```python
from build123d import *

# Parameters (mm, degrees)
SKETCH_1_W          = 80
SKETCH_1_H          = 80
EXTRUDE_1_DEPTH     = 134
SKETCH_2_R          = 40
EXTRUDE_2_DEPTH     = 1
SKETCH_3_W          = 90
SKETCH_3_H          = 90
EXTRUDE_3_DEPTH     = 10
SKETCH_4_R          = 40
EXTRUDE_4_DEPTH     = 3
SKETCH_5_R          = 20
CUT_EXTRUDE_1_DEPTH = 10
SKETCH_6_R          = 12.5
EXTRUDE_5_DEPTH     = 10
SKETCH_7_R          = 10
EXTRUDE_6_DEPTH     = 27
SKETCH_9_R          = 3.25
CUT_EXTRUDE_2_DEPTH = 10


with BuildPart() as part:
    # 草图1 → 拉伸1 (new body)
    with BuildSketch(Plane.XY):
        with Locations((40, -40)):
            Rectangle(SKETCH_1_W, SKETCH_1_H)
    extrude(amount=EXTRUDE_1_DEPTH)

    # 草图2 → 拉伸2 (add)
    with BuildSketch(Plane.XY.offset(134)):
        with Locations((40, -40)):
            Circle(SKETCH_2_R)
    extrude(amount=EXTRUDE_2_DEPTH)

    # 草图3 → 拉伸3 (add)
    with BuildSketch(Plane.XY.offset(135)):
        with Locations((40, -40)):
            Rectangle(SKETCH_3_W, SKETCH_3_H)
    extrude(amount=EXTRUDE_3_DEPTH)

    # 草图4 → 拉伸4 (add)
    with BuildSketch(Plane.XY.offset(145)):
        with Locations((40, -40)):
            Circle(SKETCH_4_R)
    extrude(amount=EXTRUDE_4_DEPTH)

    # 草图5 → 切除-拉伸1 (cut)
    with BuildSketch(Plane.XY.offset(148)):
        with Locations((40, -40)):
            Circle(SKETCH_5_R)
    extrude(amount=-CUT_EXTRUDE_1_DEPTH, mode=Mode.SUBTRACT)

    # 草图6 → 拉伸5 (add)
    with BuildSketch(Plane.XY.offset(138)):
        with Locations((40, -40)):
            Circle(SKETCH_6_R)
    extrude(amount=EXTRUDE_5_DEPTH)

    # 草图7 → 拉伸6 (add)
    with BuildSketch(Plane.XY.offset(148)):
        with Locations((40, -40)):
            Circle(SKETCH_7_R)
    extrude(amount=EXTRUDE_6_DEPTH)

    # 草图9 → 切除-拉伸2 (cut)
    with BuildSketch(Plane.XY.offset(145)):
        with Locations((75.355339059, -4.644660941)):
            Circle(SKETCH_9_R)
        with Locations((75.355339059, -75.355339059)):
            Circle(SKETCH_9_R)
        with Locations((4.644660941, -75.355339059)):
            Circle(SKETCH_9_R)
        with Locations((4.644660941, -4.644660941)):
            Circle(SKETCH_9_R)
    extrude(amount=-CUT_EXTRUDE_2_DEPTH, mode=Mode.SUBTRACT)


solid = part.part
```
Here's how the part is built. I have some questions about the finished solid (model axes, mm). A direction names the side the tool comes from. Coordinates: 2 decimals unless noted, no trailing zeros. Loops run counter-clockwise (first coordinate to the right, second up) from the corner with the lowest first, then second, coordinate; pieces in that order, holes last. Notation, with made-up numbers: M 32.25,5 L 69.25,5 A19 ccw 69.25,25 Z; hole C 35,75 d4. An arc over 180 degrees is marked long. One line per item, written item: value.
1. Please list where these lines run through material, in increasing order: probe 1 along Y at (x, z) = (40, 142); probe 2 along Z at (x, y) = (79, -67.5); probe 3 along Z at (x, y) = (31.5, -6).
Geometry says:
probe 1: y = -85 to -60, -52.5 to -27.5, -20 to 5
probe 2: z = 0 to 134, 135 to 145
probe 3: z = 0 to 148
2. Imagine slicing it at D-D (y = -69). List the corners of the cut face in (x, z) for me.
Geometry says:
outline: M -5,135 L 12.45,135 L 12.45,134 L 0,134 L 0,0 L 80,0 L 80,134 L 67.55,134 L 67.55,135 L 85,135 L 85,145 L 67.55,145 L 67.55,148 L 12.45,148 L 12.45,145 L -5,145 Z
3. Imagine slicing it at C-C (x = 43). List the corners of the cut face in (y, z) for me.
Geometry says:
outline: M -85,135 L -79.89,135 L -79.89,134 L -80,134 L -80,0 L 0,0 L 0,134 L -0.11,134 L -0.11,135 L 5,135 L 5,145 L -0.11,145 L -0.11,148 L -20.23,148 L -20.23,138 L -27.87,138 L -27.87,148 L -30.46,148 L -30.46,175 L -49.54,175 L -49.54,148 L -52.13,148 L -52.13,138 L -59.77,138 L -59.77,148 L -79.89,148 L -79.89,145 L -85,145 Z
4. Thinking about a two-plate mould opening in X: for faces 5 (the cylindrical face through (74.932, -72.133, 140.07)), 6 (the cylindrical face through (8, -64, 146)), 7 (the flat face through (39, -85, 140)), which applies, +X half, -X half, draft (parallel to the pull), parting line (faces both ways), or undercut?
Geometry says:
face 5: undercut
face 6: parting line
face 7: draft
5. Will these pins go through, and if not, where does the flat tip stop? pin 1 Ø3 at (y, z) = (-61, 114.5) entering from -X; pin 2 Ø10.5 at (x, y) = (75.36, -4.64) entering from -Z; pin 3 Ø4 at (y, z) = (-66, 128.5) entering from +X; pin 4 Ø20 at (x, y) = (69, -13.5) entering from +Z.
Geometry says:
pin 1: stops at x = 0
pin 2: stops at z = 0
pin 3: stops at x = 80
pin 4: stops at z = 148
6. On a 3-axis mill with a long thin cutter (end or side, diameter ignored), from which of +Z, -Z, +X, -X, +Y, -Y can I reach the whole of each face in a straight line? I mean faces 1 (the flat face through (8, -10, 134)), 2 (the flat face through (-1, -39, 135)), 3 (the flat face through (80, -41, 66)), 4 (the cylindrical face through (7.647, -5.889, 140.07)). Say none if no direction works.
Geometry says:
face 1: -X, +Y
face 2: none
face 3: -Z, +X, +Y, -Y
face 4: +Z
7. Imagine slicing it at B-B (x = 4). List the corners of the cut face in (y, z) for me.
Geometry says:
outline: M -85,135 L -78.54,135 L -78.54,145 L -85,145 Z; M -80,0 L 0,0 L 0,134 L -22.56,134 L -22.56,135 L -7.83,135 L -7.83,145 L -22.56,145 L -22.56,148 L -57.44,148 L -57.44,145 L -72.17,145 L -72.17,135 L -57.44,135 L -57.44,134 L -80,134 Z; M -1.46,135 L 5,135 L 5,145 L -1.46,145 Z
8. Imagine slicing it at A-A (z = 142.5). List the corners of the cut face in (x, y) for me.
Geometry says:
outline: M -5,-85 L 85,-85 L 85,5 L -5,5 Z; C 40,-40 d25; hole C 4.64,-75.36 d6.5; hole C 4.64,-4.64 d6.5; hole C 40,-40 d40; hole C 75.36,-75.36 d6.5; hole C 75.36,-4.64 d6.5
